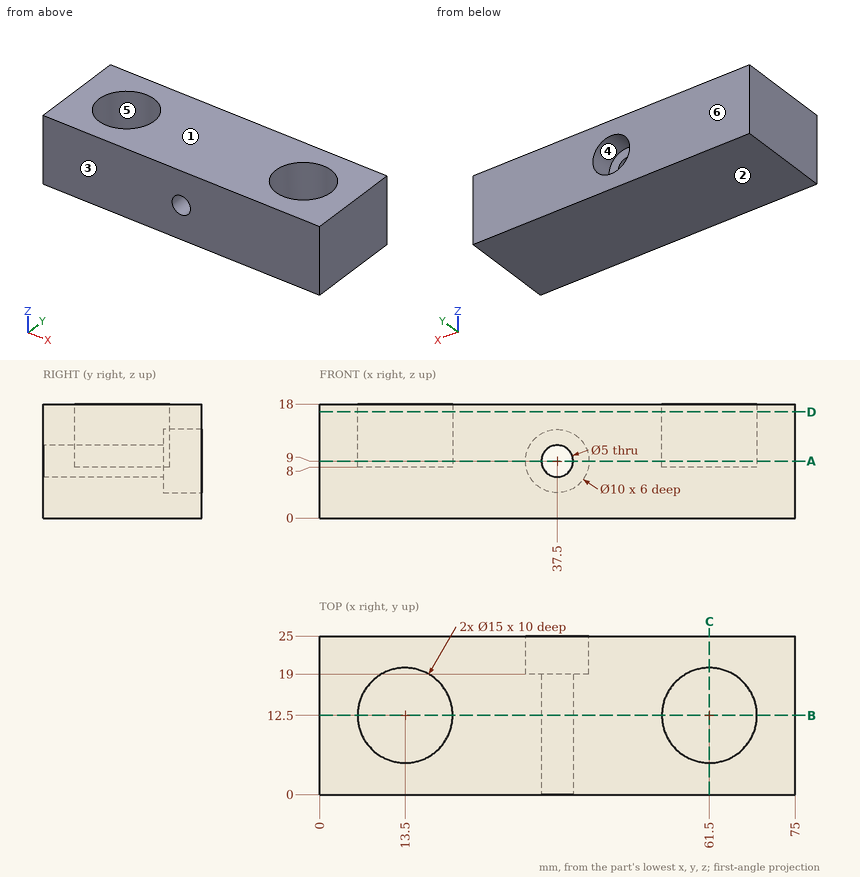
Can you work these out from the drawing? Everything is in mm from the part's minimum corner. A direction names the side the tool comes from. Coordinates: 2 decimals unless noted, no trailing zeros. Loops run counter-clockwise (first coordinate to the right, second up) from the corner with the lowest first, then second, coordinate; pieces in that order, holes last. Notation, with made-up numbers: (-1, 58.5) - (27, 58.5) arc R13 cw to (27, 78.5) - close; hole circle Ø5 at (-26, 9.25). An arc over 180 degrees is marked (long way). Use a Markdown table: item, result.
Item 1: I want a section at B-B on y = 12.5. Please give me the cut outline in (x, z).
Numbers:
| item | result |
|---|---|
| outline | (0, 0) - (75, 0) - (75, 18) - (69, 18) - (69, 8) - (54, 8) - (54, 18) - (21, 18) - (21, 8) - (6, 8) - (6, 18) - (0, 18) - close; hole circle Ø5 at (37.5, 9) |
Item 2: I want a section at C-C on x = 61.5. Please give me the cut outline in (y, z).
Numbers:
| item | result |
|---|---|
| outline | (0, 0) - (25, 0) - (25, 18) - (20, 18) - (20, 8) - (5, 8) - (5, 18) - (0, 18) - close |
Item 3: I want a section at D-D on z = 16.75. Please give me the cut outline in (x, y), and give its area (3 significant figures).
Numbers:
| item | result |
|---|---|
| outline | (0, 0) - (75, 0) - (75, 25) - (0, 25) - close; hole circle Ø15 at (13.5, 12.5); hole circle Ø15 at (61.5, 12.5) |
| area | 1,520 mm2 |
Item 4: Will these pins go through, and if not, where does the flat tip stop? pin 1 (6 mm diameter, centred on x = 11.5, y = 16, fed in from +Z); pin 2 (8 mm diameter, centred on x = 37.5, z = 9.5, fed in from +Y); pin 3 (10 mm diameter, centred on x = 46, y = 14.5, fed in from -Z).
Numbers:
| item | result |
|---|---|
| pin 1 | stops at z = 8 |
| pin 2 | stops at y = 19 |
| pin 3 | stops at z = 0 |
Item 5: For the marked faces 5 and 6, which set-ups out of +Z, -Z, +X, -X, +Y, -Y let a thin tool reach every point of the face, with its end or its side?
Numbers:
| item | result |
|---|---|
| face 5 | +Z |
| face 6 | +Z, -Z, +X, -X, +Y |
Item 6: If I drill on probe 1 along X at (y, z) = (19.25, 9.25); probe 2 along Y at (x, z) = (61.5, 13.5); probe 3 along X at (y, z) = (6.5, 13), over which ranges is the centre line in solid material (lowest first)? Write a range as from..to.
Numbers:
| item | result |
|---|---|
| probe 1 | x = 0..10.23, 16.77..32.51, 42.49..58.23, 64.77..75 |
| probe 2 | y = 0..5, 20..25 |
| probe 3 | x = 0..9, 18..57, 66..75 |
Item 7: We'd pull the mould along Z, two halves only. Please class the marked faces 1, 2, 3 and 4: released by +Z, released by -Z, zero draft, split by the parting line, or undercut.
Numbers:
| item | result |
|---|---|
| face 1 | released by +Z |
| face 2 | released by -Z |
| face 3 | zero draft |
| face 4 | undercut |
Item 8: I want a section at A-A on z = 9. Please give me the cut outline in (x, y).
Numbers:
| item | result |
|---|---|
| outline | (0, 0) - (35, 0) - (35, 19) - (32.5, 19) - (32.5, 25) - (0, 25) - close; (40, 0) - (75, 0) - (75, 25) - (42.5, 25) - (42.5, 19) - (40, 19) - close; hole circle Ø15 at (13.5, 12.5); hole circle Ø15 at (61.5, 12.5) |
